Check sheet for the modelled part. Datum: model origin and axes. Units: mm. Face numbers are marked on the shaded views. A direction names the side the tool comes from. Round coordinates to 2 decimals unless told otherwise and drop trailing zeros. Order: outer loops, then holes, each group sorted by start corner. A loop starts at its lowest first (then second) coordinate and runs counter-clockwise, first axis right, second up.
(1) Sectioned sample at B-B, the plane y = 0. Enter the section's corners in (x, z), and give its area (3 significant figures).
(2) Tool access check on the marked faces 4, 5 and 6. Record the directions out of +Z, -Z, +X, -X, +Y, -Y that give a thin tool (end or side, any length) a straight path to the whole face; none if there is none.
(3) Sectioned sample at D-D, the plane y = -53.5. Enter the section's corners in (x, z).
(4) Mould release check, pull along Y, two halves, no side actions. Record for the marked faces 1, 2 and 3: released by +Y, released by -Y, zero draft, split by the parting line, or undercut.
(5) Sectioned sample at A-A, the plane z = 14. Enter the section's corners in (x, y), and give its area (3 significant figures).
(6) Thickness scan on probe 1 along Y at (x, z) = (0, 9); probe 2 along X at (y, z) = (0, 10.5); probe 3 along Y at (x, z) = (13.5, 19). Record the ranges inside material, lowest first.
(7) Depth check by flat-ended pin: pin 1 (20 mm diameter, centred on x = 12, y = -45, fed in from +Z); pin 2 (6.5 mm diameter, centred on y = -56, z = 6, fed in from +X); pin 3 (6 mm diameter, centred on y = 9, z = 18.5, fed in from -X); pin 4 (8 mm diameter, centred on x = 2.5, y = 4, fed in from -Z). Enter the tip coordinate at first touch or a pass-through.
Autodesk Inventor part; units mm, degrees
ref_plane "YZ Plane" through (0, 0, 0) normal (1, 0, 0) x (0, 1, 0)
ref_plane "XZ Plane" through (0, 0, 0) normal (0, 1, 0) x (-1, 0, 0)
ref_plane "XY Plane" through (0, 0, 0) normal (0, 0, 1) x (1, 0, 0)
sketch "Sketch1" plane through (0, 0, 0) normal (0, 0, 1) x (1, 0, 0)
  circle A0 centre (0, 0) radius 34
  line L0 (15.5526, -72) -> (-15.5526, -72)
  line L1 (-15.5526, -72) -> (-15.5526, -49.0211)
  line L2 (-15.5526, -26.0423) -> (15.5526, -72) construction
  line L3 (15.5526, -26.0423) -> (-15.5526, -72) construction
  line L4 (-10.1666, -34) -> (10.1666, -34)
  arc A1 (-15.5526, -49.0211) -> (-26.1483, -21.7317) centre (-69.1292, -54.1216) ccw
  arc A2 (26.1483, -21.7317) -> (15.5526, -49.0211) centre (69.1292, -54.1216) ccw
  line L5 (15.5526, -49.0211) -> (15.5526, -72)
  circle A3 centre (0, 0) radius 33.2
  line L6 (-15.5526, -71.2) -> (15.5526, -71.2)
  point P0 (0, -49.0211)
  point P1 (26.1483, -21.7317)
  dimension "d0" = 68
  dimension "d1" = 38
  dimension "d2" = 0.8
  dimension "d3" = 0.8
extrude "Extrusion1" add sketch "Sketch1" along normal blind 0.8 contours A0 A2 L5 L6 L1 A1 | A3
extrude "Extrusion2" add sketch "Sketch1" along normal blind 25 contours L6 L5 L0 L1
extrude "Extrusion3" add sketch "Sketch1" along normal blind 35 contours A0
sketch "Sketch2" plane through (-15.5526, -72, 0) normal (0, -1, 0) x (1, 0, 0)
  line L0 (31.1053, 25) -> (0, 25)
  arc A0 (5.7113, 25) -> (25.3939, 25) centre (15.5526, 25) ccw
  line L1 (5.7113, 25) -> (25.3939, 25)
  point P0 (15.5526, 0)
extrude "Extrusion4" cut sketch "Sketch2" against normal blind 2
sketch "Sketch3" plane through (0, 0, 0.8) normal (0, 0, 1) x (1, 0, 0)
  line L0 (-9.8413, -71.2) -> (9.8413, -71.2)
  line L1 (-1.3972, -33.6906) -> (1.3972, -33.6906)
  line L2 (1.3972, -33.6906) -> (1.3972, -71.2)
  line L3 (1.3972, -71.2) -> (-1.3972, -71.2)
  line L4 (-1.3972, -71.2) -> (-1.3972, -33.6906)
  line L5 (-1.3972, -33.6906) -> (1.3972, -71.2) construction
  line L6 (1.3972, -33.6906) -> (-1.3972, -71.2) construction
  point P0 (0, 0)
  point P1 (0, -52.4453)
extrude "Extrusion5" add sketch "Sketch3" along normal blind 8
sketch "Sketch4" plane through (1.3972, -71.2, 0.8) normal (1, 0, 0) x (0, 0, -1)
  point P0 (0.8, 71.2)
sketch "Sketch5" plane through (1.3972, -71.2, 0.8) normal (1, 0, 0) x (0, 0, -1)
  line L0 (-12.1, 0) -> (-14.4584, 0)
  arc A0 (-8.7861, 0) -> (-8.7861, 37.2287) centre (-31.8736, 18.6144) ccw
  line L1 (-8.7861, 37.374) -> (-8.7861, 37.374)
  line L2 (-8, 37.2287) -> (0, 37.2287)
  line L3 (-8.7861, 37.374) -> (-8.7861, 0)
  point P0 (0.8, 71.2)
  point P1 (-25, 0)
  point P2 (-24.2, 37.2287)
extrude "Extrusion6" cut sketch "Sketch5" against normal up to surface (2.7945 mm away)
sketch "Sketch7" plane through (0, 0, 35) normal (0, 0, 1) x (1, 0, 0)
  line L0 (-14, -28.6906) -> (14, -28.6906)
  line L1 (14, -28.6906) -> (14, -38.6906)
  line L2 (14, -38.6906) -> (-14, -38.6906)
  line L3 (-14, -38.6906) -> (-14, -28.6906)
  line L4 (-1.3972, -33.6906) -> (1.3972, -33.6906)
  line L5 (-14, -28.6906) -> (14, -38.6906) construction
  line L6 (14, -28.6906) -> (-14, -38.6906) construction
  point P0 (0, 0)
  point P1 (0, -33.6906)
  dimension "d23" = 28
  dimension "d24" = 10
extrude "Extrusion8" cut sketch "Sketch7" against normal blind 12
properties part number "my_portafilter_holder"
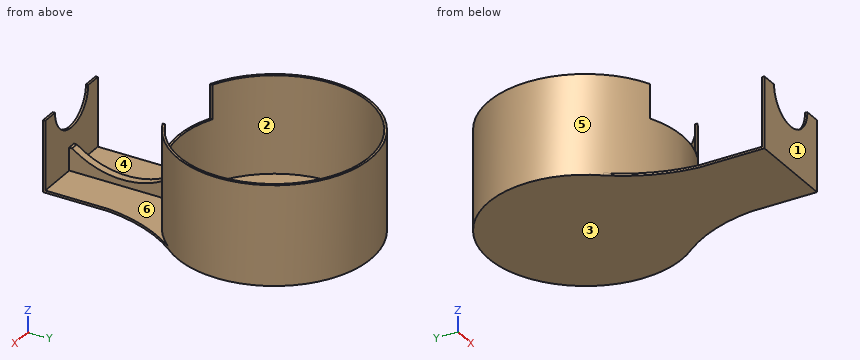
Derived:
1. outline: (-34, 0) - (34, 0) - (34, 35) - (33.2, 35) - (33.2, 0.8) - (-33.2, 0.8) - (-33.2, 35) - (-34, 35) - close
1. area: 109 mm2
2. face 4: +Z, -X
2. face 5: +Z
2. face 6: +Z, +X
3. outline: (-15.55, 0) - (15.55, 0) - (15.55, 0.8) - (1.4, 0.8) - (1.4, 3.03) - (-1.4, 3.03) - (-1.4, 0.8) - (-15.55, 0.8) - close
4. face 1: released by -Y
4. face 2: undercut
4. face 3: zero draft
5. outline: circle Ø68 at (0, 0); (-15.55, -72) - (15.55, -72) - (15.55, -71.2) - (-15.55, -71.2) - close; hole circle Ø66.4 at (0, 0)
5. area: 194 mm2
6. probe 1: y = -72 to -71.2, -34 to -33.2, 33.2 to 34
6. probe 2: x = -34 to -33.2, 33.2 to 34
6. probe 3: y = -72 to -71.2, -31.2 to -30.33, 30.33 to 31.2
7. pin 1: stops at z = 0.8
7. pin 2: stops at x = 1.4
7. pin 3: stops at x = -33.47
7. pin 4: stops at z = 0
